Source: CAD feature listing. Evaluate the final solid. Frame: model axes, mm. A direction names the side the tool comes from. Coordinates: 2 decimals unless noted, no trailing zeros. Loops run counter-clockwise (first coordinate to the right, second up) from the corner with the lowest first, then second, coordinate; pieces in that order, holes last.
```python
from build123d import *

# Parameters (mm, degrees)
SKETCH_1_R          = 13.1
EXTRUDE_1_DEPTH     = 35
SKETCH_2_R          = 19.270653491
SKETCH_2_R_2        = 8
CUT_EXTRUDE_1_DEPTH = 1
SKETCH_3_R          = 17.55104744
SKETCH_3_R_2        = 10.25
CUT_EXTRUDE_2_DEPTH = 0.1
FILLET_1_R          = 0.5


with BuildPart() as part:
    # Эскиз1 → Бобышка-Вытянуть1 (new body)
    with BuildSketch(Plane(origin=(0, 0, 0), x_dir=(1, 0, 0), z_dir=(0, 1, 0))):
        with Locations(Location((0, 0, 0), (0, 0, 270))):
            Circle(SKETCH_1_R)
    extrude(amount=EXTRUDE_1_DEPTH)

    # Эскиз2 → Вырез-Вытянуть1 (cut)
    with BuildSketch(Plane(origin=(0, 35, 0), x_dir=(1, 0, 0), z_dir=(0, 1, 0))):
        Circle(SKETCH_2_R)
        with Locations(Location((0, 0, 0), (0, 0, 270))):
            Circle(SKETCH_2_R_2, mode=Mode.SUBTRACT)
    extrude(amount=-CUT_EXTRUDE_1_DEPTH, mode=Mode.SUBTRACT)

    # Эскиз3 → Вырез-Вытянуть2 (cut)
    with BuildSketch(Plane.XZ):
        Circle(SKETCH_3_R)
        with Locations(Location((0, 0, 0), (0, 0, 270))):
            Circle(SKETCH_3_R_2, mode=Mode.SUBTRACT)
    extrude(amount=-CUT_EXTRUDE_2_DEPTH, mode=Mode.SUBTRACT)

    # Скругление1
    fillet_1_edges = [part.edges().sort_by_distance(p)[0] for p in [
        (0, 0.1, -13.1),
        (0, 34, -13.1),
    ]]
    fillet(fillet_1_edges, radius=FILLET_1_R)


solid = part.part
```
Q1. Reachability of faces 1 (the flat face through (-0.2, 34, 8.2)), 2 (the cylindrical face through (11.046, 16.82, 7.042)), 3 (the flat face through (3, 0.1, -10)) from +Z, -Z, +X, -X, +Y, -Y: full face, straight path, thin tool, end or side. Return the list, or none.
Q2. First-contact query: pin 1 Ø6 at (y, z) = (7, -3) entering from +X; pin 2 Ø10 at (x, y) = (5.5, 13.5) entering from +Z; pin 3 Ø1.5 at (y, z) = (7, 3) entering from -X; pin 4 Ø1.5 at (y, z) = (18, 2) entering from +X. Flat tips, straight axial feed; report the tip coordinate or a pass-through.
Q3. Material intervals for line 1 along Y through (x, z) = (7, 9.25); line 2 along X through (y, z) = (14, 0); line 3 along X through (y, z) = (9, -5.5), sorted ascending.
Q4. Section query A-A on y = 27. Return the cut outline in (x, z).
Resolved:
1. face 1: +Y
1. face 2: +Y, -Y
1. face 3: -Y
2. pin 1: stops at x = 13.1
2. pin 2: stops at z = 13.09
2. pin 3: stops at x = -12.91
2. pin 4: stops at x = 13.04
3. line 1: y = 0.1 to 34
3. line 2: x = -13.1 to 13.1
3. line 3: x = -11.89 to 11.89
4. outline: circle Ø26.2 at (0, 0)
